Can you work these out from the model? Positions are in its coordinate system, mm. A direction names the side the tool comes from. Round coordinates to 2 decimals unless told otherwise and drop trailing zeros. Write each loop counter-clockwise with the first axis right and the second up, starting at its lowest first coordinate (ties: lowest second). Pieces come first, ordered by that corner, then holes.
Q1. We'd pull the mould along X, two halves only. Please class faces 4 (the flat face through (0, -1, 5)), 5 (the cylindrical face through (5.95, 3.16, 3.6)), 6 (the flat face through (105, 6.4, 3)): +X half, -X half, draft (parallel to the pull), parting line (faces both ways), or undercut.
Q2. For faces 1 (the flat face through (70, 3, 5)), 2 (the cylindrical face through (65.998, 2.141, 3.519)), 3 (the cylindrical face through (15.338, 3.155, 4.073)), which set-ups out of +Z, -Z, +X, -X, +Y, -Y let a thin tool reach every point of the face, with its end or its side?
Q3. If we section it at D-D (x = 115): Please give me the cut outline in (y, z) (3 decimals), plus the area to 3 significant figures.
Q4. If we section it at A-A (x = 65): Please give me the cut outline in (y, z) (3 decimals), plus the area to 3 significant figures.
Q5. I'm going to push flat-ended pins straight in: pin 1 Ø3 at (x, z) = (22, 6.5) entering from +Y; pin 2 Ø3 at (y, z) = (4.5, 2.5) entering from -X (3 decimals); pin 3 Ø4 at (y, z) = (4, 6.5) entering from +X. Where does each tip first touch, or does it pass through?
Q6. Please list where these lines run through material, in increasing order: line 1 along X through (y, z) = (-0.9, 3) (3 decimals); line 2 along Z through (x, y) = (65, 0.5) (3 decimals); line 3 along Y through (x, z) = (80, 3.75).
Q7. If we section it at B-B (y = 2.5): Please give me the cut outline in (x, z) (3 decimals), plus the area to 3 significant figures.
Q8. If we section it at C-C (z = 3): Give the number of separate pieces and of enclosed holes in the cut face, plus the area to 3 significant figures.
from build123d import *

# Parameters (mm, degrees)
SKETCH2_W           = 40
SKETCH2_H           = 10
BOSS_EXTRUDE1_DEPTH = 2
SKETCH2_3_W         = 20
SKETCH2_3_H         = 10
SKETCH2_3_R         = 1.125
BOSS_EXTRUDE2_DEPTH = 2
SKETCH2_4_R         = 1.125
BOSS_EXTRUDE3_DEPTH = 6.4
SKETCH4_W           = 10
SKETCH4_H           = 10
SKETCH4_R           = 1.125
BOSS_EXTRUDE4_DEPTH = 6.4
SKETCH4_2_R         = 1.125
CUT_EXTRUDE2_DEPTH  = 62.163387741


with BuildPart() as part:
    # Sketch2 → Boss-Extrude1 (new body)
    with BuildSketch(Plane(origin=(0, 0, 0), x_dir=(1, 0, 0), z_dir=(0, 1, 0))):
        with Locations((40, -5)):
            Rectangle(SKETCH2_W, SKETCH2_H)
    boss_extrude1 = extrude(amount=-BOSS_EXTRUDE1_DEPTH)

    # Sketch2_3 → Boss-Extrude2 (add)
    # profile 1 of 3: a face of its own
    with BuildSketch(Plane(origin=(0, 0, 0), x_dir=(1, 0, 0), z_dir=(0, 1, 0))):
        with Locations((10, -5)):
            Rectangle(SKETCH2_3_W, SKETCH2_3_H)
        with Locations((15, -3)):
            Circle(SKETCH2_3_R, mode=Mode.SUBTRACT)
        with Locations((5, -3)):
            Circle(SKETCH2_3_R, mode=Mode.SUBTRACT)
    # profile 2 of 3: a face of its own
    with BuildSketch(Plane(origin=(0, 0, 0), x_dir=(1, 0, 0), z_dir=(0, 1, 0))):
        with Locations((15, -3)):
            Circle(SKETCH2_3_R)
    # profile 3 of 3: a face of its own
    with BuildSketch(Plane(origin=(0, 0, 0), x_dir=(1, 0, 0), z_dir=(0, 1, 0))):
        with Locations((5, -3)):
            Circle(SKETCH2_3_R)
    boss_extrude2 = extrude(amount=-BOSS_EXTRUDE2_DEPTH)

    # Sketch2_4 → Boss-Extrude3 (add)
    with BuildSketch(Plane(origin=(0, 0, 0), x_dir=(1, 0, 0), z_dir=(0, 1, 0))):
        with Locations(Location((15, -3, 0), (0, 0, 270))):
            Circle(SKETCH2_4_R)
        with Locations(Location((5, -3, 0), (0, 0, 270))):
            Circle(SKETCH2_4_R)
    boss_extrude3 = extrude(amount=BOSS_EXTRUDE3_DEPTH)

    # Sketch4 → Boss-Extrude4 (add)
    with BuildSketch(Plane(origin=(0, 0, 0), x_dir=(1, 0, 0), z_dir=(0, 1, 0))):
        with Locations((55, -5)):
            Rectangle(SKETCH4_W, SKETCH4_H)
        with Locations(Location((55, -3, 0), (0, 0, 270))):
            Circle(SKETCH4_R, mode=Mode.SUBTRACT)
    boss_extrude4 = extrude(amount=BOSS_EXTRUDE4_DEPTH)

    # Sketch4_2 → Cut-Extrude2 (cut, through all)
    with BuildSketch(Plane(origin=(0, 0, 0), x_dir=(1, 0, 0), z_dir=(0, 1, 0))):
        with Locations(Location((55, -3, 0), (0, 0, 270))):
            Circle(SKETCH4_2_R)
    cut_extrude2 = extrude(amount=-CUT_EXTRUDE2_DEPTH, mode=Mode.SUBTRACT)

    # Mirror2: Boss-Extrude1, Boss-Extrude2, Boss-Extrude3, Boss-Extrude4, Cut-Extrude2 across plane
    add(boss_extrude1.mirror(Plane(origin=(60, -2, 0), x_dir=(0, 0, 1), z_dir=(-1, 0, 0))))
    add(boss_extrude2.mirror(Plane(origin=(60, -2, 0), x_dir=(0, 0, 1), z_dir=(-1, 0, 0))))
    add(boss_extrude3.mirror(Plane(origin=(60, -2, 0), x_dir=(0, 0, 1), z_dir=(-1, 0, 0))))
    add(boss_extrude4.mirror(Plane(origin=(60, -2, 0), x_dir=(0, 0, 1), z_dir=(-1, 0, 0))))
    add(cut_extrude2.mirror(Plane(origin=(60, -2, 0), x_dir=(0, 0, 1), z_dir=(-1, 0, 0))), mode=Mode.SUBTRACT)


solid = part.part
A:
1. face 4: -X half
1. face 5: undercut
1. face 6: draft
2. face 1: +Z, -Z, +Y
2. face 2: +Y, -Y
2. face 3: +Y
3. outline: (-2, 0) - (0, 0) - (0, 1.875) - (6.4, 1.875) - (6.4, 4.125) - (0, 4.125) - (0, 10) - (-2, 10) - close
3. area: 34.4 mm2
4. outline: (-2, 0) - (6.4, 0) - (6.4, 1.875) - (-2, 1.875) - close; (-2, 4.125) - (6.4, 4.125) - (6.4, 10) - (-2, 10) - close
4. area: 65.1 mm2
5. pin 1: stops at y = 0
5. pin 2: stops at x = 3.875
5. pin 3: stops at x = 70
6. line 1: x = 0 to 53.875, 56.125 to 63.875, 66.125 to 120
6. line 2: z = 0 to 1.875, 4.125 to 10
6. line 3: y = -2 to 0
7. outline: circle Ø2.25 at (5, 3); circle Ø2.25 at (15, 3); (50, 0) - (70, 0) - (70, 10) - (50, 10) - close; circle Ø2.25 at (105, 3); circle Ø2.25 at (115, 3); hole circle Ø2.25 at (55, 3); hole circle Ø2.25 at (65, 3)
7. area: 208 mm2
8. separate pieces: 3
8. enclosed holes: 0
8. area: 388 mm2
